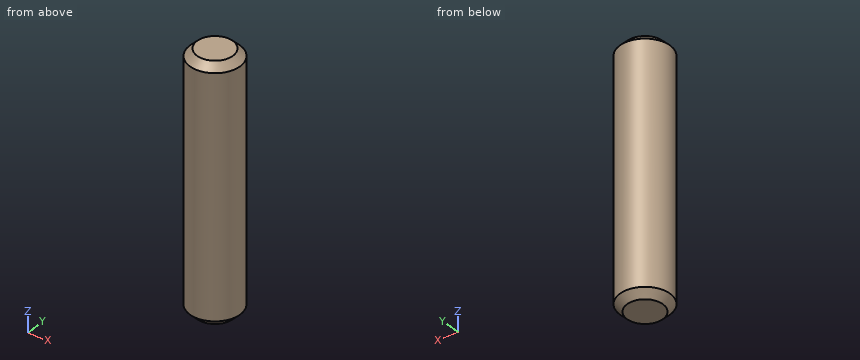
```python
from build123d import *

# Parameters (mm, degrees)
SKETCH2_R           = 7
BOSS_EXTRUDE1_DEPTH = 35
CHAMFER1_SIZE       = 2
CHAMFER2_SIZE       = 2


with BuildPart() as part:
    # Sketch2 → Boss-Extrude1 (new body, symmetric)
    with BuildSketch(Plane.XY):
        Circle(SKETCH2_R)
    extrude(amount=BOSS_EXTRUDE1_DEPTH, both=True)

    # Chamfer1
    chamfer1_edges = [part.edges().sort_by_distance(p)[0] for p in [
        (-7, 0, -35),
    ]]
    chamfer(chamfer1_edges, length=CHAMFER1_SIZE)

    # Chamfer2
    chamfer2_edges = [part.edges().sort_by_distance(p)[0] for p in [
        (-7, 0, 35),
    ]]
    chamfer(chamfer2_edges, length=CHAMFER2_SIZE)


solid = part.part
```
Model file for the job. Use its own axes, mm. Give positions to 0.01 mm unless a question says otherwise; leave off trailing zeros. Order: outer loops, then holes, each group sorted by start corner. A loop starts at its lowest first (then second) coordinate and runs counter-clockwise, first axis right, second up.
1) Pin check, flat tips, straight feed: pin 1 (1 mm diameter, centred on y = 1, z = -9, fed in from +X); pin 2 (1 mm diameter, centred on y = -2, z = 10, fed in from -X); pin 3 (3 mm diameter, centred on x = -5.5, z = 9.5, fed in from -Y). Stop position of each tip, or through.
2) Saw through at A-A, the plane z = 29.5. Write the cut outline in (x, y).
3) Wall check: probe 1 along X at (y, z) = (-1, -12); probe 2 along Y at (x, z) = (-4.75, 5); probe 3 along Y at (x, z) = (-0.75, 12.5). Give the ranges that are in metal, low to high.
Computed:
1. pin 1: stops at x = 6.98
1. pin 2: stops at x = -6.84
1. pin 3: stops at y = -5.74
2. outline: circle Ø14 at (0, 0)
3. probe 1: x = -6.93 to 6.93
3. probe 2: y = -5.14 to 5.14
3. probe 3: y = -6.96 to 6.96
